Source: three-view drawing plus pictorial views. Frame: mm from the lowest corner of the part. A direction names the side the tool comes from. Coordinates: 2 decimals unless noted, no trailing zeros. Order: outer loops, then holes, each group sorted by start corner. A loop starts at its lowest first (then second) coordinate and runs counter-clockwise, first axis right, second up. Notation, with made-up numbers: (31.5, 81) -> (41.5, 81) arc R11 cw to (41.5, 94) -> close; hole circle Ø6 at (76.5, 38). An arc over 180 degrees is marked (long way). Use CSV: the item, a comma, the result in double quotes. Start each with the question number.
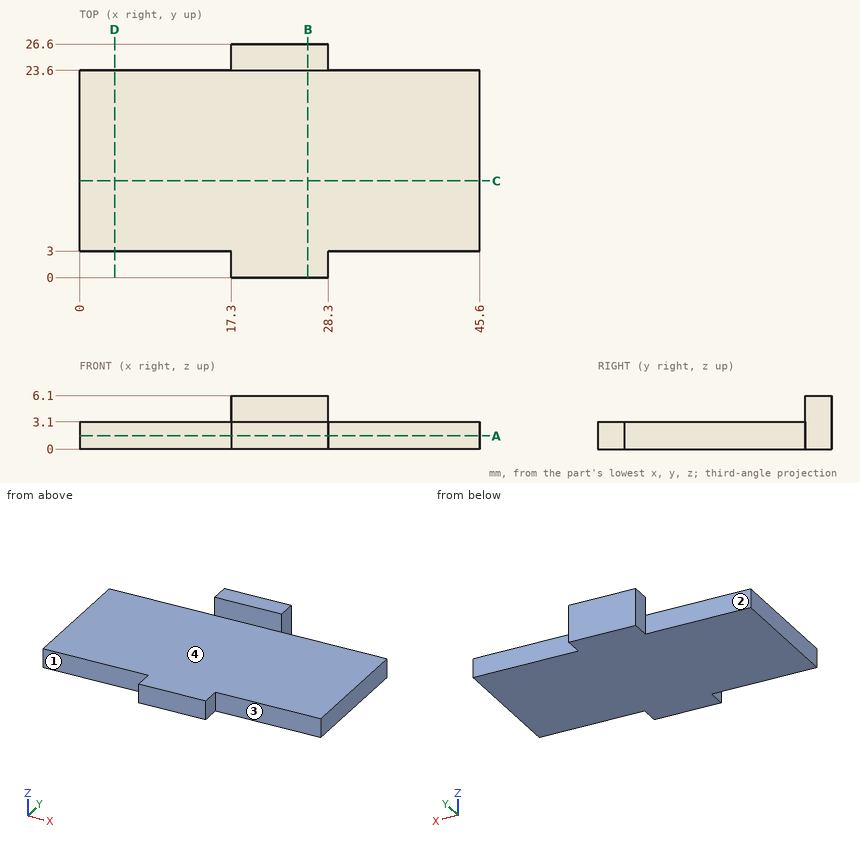
1. Section C-C on y = 11. Return loops of the section in (x, z), then the cut area to 3 significant figures.
2. Contact query for flat-ended pins moving along their axis: P1, Ø2.5, axis at y = 25.5, z = 3, coming from the -X side; P2, Ø2.5, axis at x = 36, z = 1, coming from the -Y side; P3, Ø1, axis at x = 32, z = 2, coming from the +Y side. Output: stop coordinate, or through.
3. Section D-D on x = 4. Return loops of the section in (y, z).
4. Access query for the marked faces 1, 2, 3 and 4. Directions: +Z, -Z, +X, -X, +Y, -Y. A direction counts if a zero-diameter tool reaches every point of the face in a straight line with its end or side. Return the directions, or none.
5. Material intervals for line 1 along Z through (x, y) = (13.5, 17.25); line 2 along Y through (x, z) = (5.5, 0.5); line 3 along Y through (x, z) = (20, 4.25), sorted ascending.
6. Section A-A on z = 1.5. Return loops of the section in (x, y).
7. Section B-B on x = 26. Return loops of the section in (y, z).
Values follow:
1,outline,"(0, 0) -> (45.6, 0) -> (45.6, 3.1) -> (0, 3.1) -> close"
1,area,"141 mm2"
2,P1,"stops at x = 17.3"
2,P2,"stops at y = 3"
2,P3,"stops at y = 23.6"
3,outline,"(3, 0) -> (23.6, 0) -> (23.6, 3.1) -> (3, 3.1) -> close"
4,face 1,"+Z, -Z, -X, -Y"
4,face 2,"+Z, -Z, -X, +Y"
4,face 3,"+Z, -Z, +X, -Y"
4,face 4,"+Z, +X, -X, -Y"
5,line 1,"z = 0 to 3.1"
5,line 2,"y = 3 to 23.6"
5,line 3,"y = 23.6 to 26.6"
6,outline,"(0, 3) -> (17.3, 3) -> (17.3, 0) -> (28.3, 0) -> (28.3, 3) -> (45.6, 3) -> (45.6, 23.6) -> (28.3, 23.6) -> (28.3, 26.6) -> (17.3, 26.6) -> (17.3, 23.6) -> (0, 23.6) -> close"
7,outline,"(0, 0) -> (26.6, 0) -> (26.6, 6.1) -> (23.6, 6.1) -> (23.6, 3.1) -> (0, 3.1) -> close"
